from build123d import *
from OCP.BRepAlgoAPI import BRepAlgoAPI_Cut
from OCP.TopTools import TopTools_ListOfShape

# Parameters (mm, degrees)
SKETCH1_W           = 78.232
SKETCH1_H           = 90.17
BOSS_EXTRUDE1_DEPTH = 3.175
FILLET1_R           = 3.175
SKETCH2_W           = 2.032
SKETCH2_H           = 50.8
SKETCH2_W_2         = 38.1
SKETCH2_H_2         = 2.032
BOSS_EXTRUDE2_DEPTH = 5.08
FILLET3_R           = 0.508
CUT_EXTRUDE1_DEPTH  = 63.761267046
CHAMFER2_SIZE       = 0.762


with BuildPart() as part:
    # Sketch1 → Boss-Extrude1 (new body)
    with BuildSketch(Plane(origin=(0, 0, 0), x_dir=(1, 0, 0), z_dir=(0, 1, 0))):
        Rectangle(SKETCH1_W, SKETCH1_H)
        with BuildLine():
            Line((-5.334, 7.493), (5.588, 7.493))
            ThreePointArc((5.588, 7.493), (7.756025612, 8.391025612), (6.858, 6.223))
            Line((6.858, 6.223), (6.858, -6.096))
            ThreePointArc((6.858, -6.096), (7.756025612, -8.264025612), (5.588, -7.366))
            Line((5.588, -7.366), (-5.334, -7.366))
            ThreePointArc((-5.334, -7.366), (-7.502025612, -8.264025612), (-6.604, -6.096))
            Line((-6.604, -6.096), (-6.604, 6.223))
            ThreePointArc((-6.604, 6.223), (-7.502025612, 8.391025612), (-5.334, 7.493))
        make_face(mode=Mode.SUBTRACT)
    extrude(amount=BOSS_EXTRUDE1_DEPTH)

    # Fillet1
    fillet1_edges = [part.edges().sort_by_distance(p)[0] for p in [
        (-39.116, 1.5875, -45.085),
        (39.116, 1.5875, -45.085),
        (39.116, 1.5875, 45.085),
        (-39.116, 1.5875, 45.085),
    ]]
    fillet(fillet1_edges, radius=FILLET1_R)


with BuildPart() as boss_extrude2_tool:
    # Sketch2 → Boss-Extrude2 (new body)
    with BuildSketch(Plane(origin=(0, 3.175, 0), x_dir=(1, 0, 0), z_dir=(0, 1, 0))):
        Polygon((19.049995564, -47.117005476), (19.049995755, -45.085005476), (-19.050004245, -45.085001889), (-19.050004436, -47.117001889), align=None)
        with Locations((-40.132001661, 0)):
            Rectangle(SKETCH2_W, SKETCH2_H)
        with Locations((0, 46.101)):
            Rectangle(SKETCH2_W_2, SKETCH2_H_2)
        with Locations((40.132001661, 0)):
            Rectangle(SKETCH2_W, SKETCH2_H)
    extrude(amount=-BOSS_EXTRUDE2_DEPTH)


with BuildPart() as part_1:
    add(part.part)


with BuildPart() as part_2:
    # Boss-Extrude2: joined with boss_extrude2_tool
    add(part_1.part.fuse(boss_extrude2_tool.part, tol=0.00001))

    # Fillet3
    fillet3_edges = [part_2.edges().sort_by_distance(p)[0] for p in [
        (19.05, 1.5875, -45.085),
        (-19.05, 1.5875, -45.085),
        (-19.05, 0.635, -47.117),
        (19.05, 0.635, -47.117),
        (-39.116001661, 1.5875, 25.4),
        (-39.116001661, 1.5875, -25.4),
        (-41.148001661, 0.635, 25.4),
        (-41.148001661, 0.635, -25.4),
        (39.116001661, 1.5875, 25.4),
        (39.116001661, 1.5875, -25.4),
        (41.148001661, 0.635, -25.4),
        (41.148001661, 0.635, 25.4),
        (19.049995755, 1.5875, 45.085005476),
        (-19.050004245, 1.5875, 45.085001889),
        (19.049995564, 0.635, 47.117005476),
        (-19.050004436, 0.635, 47.117001889),
    ]]
    fillet(fillet3_edges, radius=FILLET3_R)


with BuildPart() as cut_extrude1_tool:
    # Sketch3 → Cut-Extrude1 (new, through all)
    with BuildSketch(Plane(origin=(0, 3.175, 0), x_dir=(1, 0, 0), z_dir=(0, 1, 0))):
        with BuildLine():
            Line((-39.116, 36.5), (-39.116, 33.5))
            ThreePointArc((-39.116, 33.5), (-37.616, 35), (-39.116, 36.5))
        make_face()
        with BuildLine():
            Line((-27.5, 45.085), (-30.5, 45.085))
            ThreePointArc((-30.5, 45.085), (-29, 43.585), (-27.5, 45.085))
        make_face()
        with BuildLine():
            Line((27.499999809, 45.084997268), (30.499999809, 45.084997268))
            ThreePointArc((30.499999809, 45.084997268), (28.999999809, 43.584997268), (27.499999809, 45.084997268))
        make_face()
        with BuildLine():
            Line((39.115998859, 36.499996315), (39.115998859, 33.499996315))
            ThreePointArc((39.115998859, 33.499996315), (37.615998859, 34.999996315), (39.115998859, 36.499996315))
        make_face()
        with BuildLine():
            Line((39.115998859, -33.499996315), (39.115998859, -36.499996315))
            ThreePointArc((39.115998859, -36.499996315), (37.615998859, -34.999996315), (39.115998859, -33.499996315))
        make_face()
        with BuildLine():
            Line((30.499999809, -45.084997268), (27.499999809, -45.084997268))
            ThreePointArc((27.499999809, -45.084997268), (28.999999809, -43.584997268), (30.499999809, -45.084997268))
        make_face()
        with BuildLine():
            Line((-27.5, -45.085), (-30.5, -45.085))
            ThreePointArc((-30.5, -45.085), (-29, -43.585), (-27.5, -45.085))
        make_face()
        with BuildLine():
            Line((-39.116, -36.5), (-39.116, -33.5))
            ThreePointArc((-39.116, -33.5), (-37.616, -35), (-39.116, -36.5))
        make_face()
    extrude(amount=-CUT_EXTRUDE1_DEPTH)


with BuildPart() as part_3:
    add(part_2.part)

    # Cut-Extrude1: cut by cut_extrude1_tool, with a tolerance
    cut_extrude1_stock = TopTools_ListOfShape()
    cut_extrude1_stock.Append(part_3.part.wrapped)
    cut_extrude1_tools = TopTools_ListOfShape()
    cut_extrude1_tools.Append(cut_extrude1_tool.part.wrapped)
    cut_extrude1_cut = BRepAlgoAPI_Cut()
    cut_extrude1_cut.SetArguments(cut_extrude1_stock)
    cut_extrude1_cut.SetTools(cut_extrude1_tools)
    cut_extrude1_cut.SetFuzzyValue(0.00001)
    cut_extrude1_cut.Build()
    add(Compound.cast(cut_extrude1_cut.Shape()).solids(), mode=Mode.REPLACE)

    # Chamfer2
    chamfer2_edges = [part_3.edges().sort_by_distance(p)[0] for p in [
        (-7.502025612, 3.175, -8.391025612),
        (-6.604, 3.175, -0.0635),
        (-7.502025612, 3.175, 8.264025612),
        (0.127, 3.175, 7.366),
        (7.756025612, 3.175, 8.264025612),
        (6.858, 3.175, -0.0635),
        (7.756025612, 3.175, -8.391025612),
        (0.127, 3.175, -7.493),
    ]]
    chamfer(chamfer2_edges, length=CHAMFER2_SIZE)


solid = part_3.part
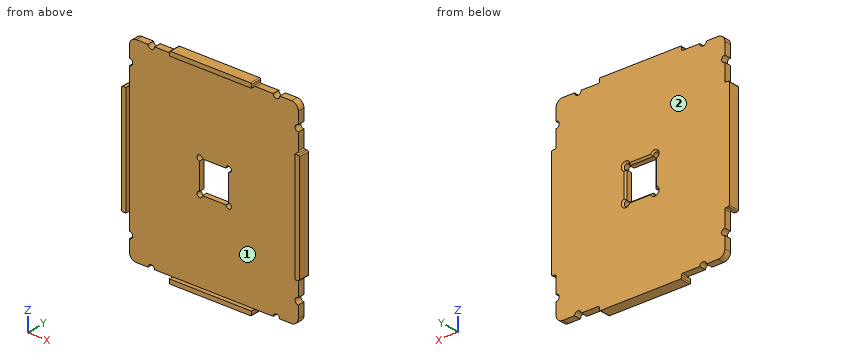
The listing builds one solid part. Answer for the finished solid, in the listing's coordinates (mm). Face numbers are marked on the shaded views. Give positions to 0.01 mm unless a question says otherwise; leave off trailing zeros. Loops run counter-clockwise (first coordinate to the right, second up) from the corner with the lowest first, then second, coordinate; pieces in that order, holes last. Notation, with made-up numbers: (60.25, 84.5) - (116.25, 84.5) arc R7 ccw to (116.25, 88.5) - close; hole circle Ø3 at (29, 63). An arc over 180 degrees is marked (long way). Write each question's results on one line, items separated by ' | '.
1. Consider probe 1 along X at (y, z) = (0.3, 5); probe 2 along Z at (x, y) = (13, -0.7) (3 decimals); probe 3 along X at (y, z) = (-0.6, -21.5). Determine where each line is inside the solid, lowest interval first. Write a range as from..to.
Resolved:
probe 1: x = -41.15..-6.6, 6.86..41.15 | probe 2: z = -47.117..-45.085, 45.085..47.117 | probe 3: x = -41.15..-39.12, 39.12..41.15
2. Find section D-D, the plane x = 29. Write down the section's boundary in (y, z) (3 decimals), then the cut area to 3 significant figures.
Resolved:
outline: (0, -43.585) - (3.175, -43.585) - (3.175, 43.585) - (0, 43.585) - close | area: 277 mm^2
3. For a pull along Z with two mould halves and no side action, classify the marked faces 1 and 2 as +Z half, -Z half, draft (parallel to the pull), parting line (faces both ways), or undercut.
Resolved:
face 1: undercut | face 2: draft
4. Find section B-B, the plane x = 14. Write down the section's boundary in (y, z) (3 decimals).
Resolved:
outline: (-1.905, -47.117) - (3.175, -47.117) - (3.175, 47.117) - (-1.905, 47.117) - (-1.905, 45.085) - (0, 45.085) - (0, -45.085) - (-1.905, -45.085) - close
5. Flat-ended cylindrical pins translate along their axes: P1, Ø2, axis at y = 2.5, z = 32.5, coming from the +X side; P2, Ø2, axis at x = 31, y = 2.5, coming from the +Z side (3 decimals); P3, Ø2.5, axis at y = 1, z = 40, coming from the -X side. Find the tip coordinate at first contact, or state that the pin passes through.
Resolved:
P1: stops at x = 39.12 | P2: stops at z = 45.085 | P3: stops at x = -39.12
6. Find section C-C, the plane z = 32. Write down the section's boundary in (x, y) (3 decimals), then the cut area to 3 significant figures.
Resolved:
outline: (-39.116, 0) - (39.116, 0) - (39.116, 3.175) - (-39.116, 3.175) - close | area: 248 mm^2
7. Find section A-A, the plane z = 1. Write down the section's boundary in (x, y) (3 decimals), then the cut area to 3 significant figures.
Resolved:
outline: (-41.148, -1.905) - (-39.116, -1.905) - (-39.116, 0) - (-6.604, 0) - (-6.604, 2.413) - (-7.366, 3.175) - (-41.148, 3.175) - close; (6.858, 0) - (39.116, 0) - (39.116, -1.905) - (41.148, -1.905) - (41.148, 3.175) - (7.62, 3.175) - (6.858, 2.413) - close | area: 226 mm^2
